```python
from build123d import *

# Parameters (mm, degrees)
ESTRUSIONE_ESTRUSIONE9_DEPTH = 50
SMUSSO1_SIZE                 = 0.75


with BuildPart() as part:
    # Schizzo16 → Estrusione-Estrusione9 (new body)
    with BuildSketch(Plane(origin=(0, 0, 0), x_dir=(0, 0, -1), z_dir=(1, 0, 0))):
        Polygon((0, 0), (5, 0), (5, 6), (43, 6), (43, 0), (48, 0), (48, 9), (0, 9), align=None)
    extrude(amount=ESTRUSIONE_ESTRUSIONE9_DEPTH)

    # Smusso1
    smusso1_edges = [part.edges().sort_by_distance(p)[0] for p in [
        (0, 4.5, 0),
        (50, 4.5, -48),
        (50, 4.5, 0),
        (0, 4.5, -48),
    ]]
    chamfer(smusso1_edges, length=SMUSSO1_SIZE)


solid = part.part
```
The listing builds one solid part. Answer for the finished solid, in the listing's coordinates (mm). A direction names the side the tool comes from. Coordinates: 2 decimals unless noted, no trailing zeros. Loops run counter-clockwise (first coordinate to the right, second up) from the corner with the lowest first, then second, coordinate; pieces in that order, holes last. Notation, with made-up numbers: (42, -16) - (78, -16) arc R18 ccw to (78, 11) - close; hole circle Ø5 at (76.5, 46.25). An arc over 180 degrees is marked (long way). Use a Markdown table: item, result. Add a question column.
1) The part is cut by section A-A, the plane y = 3. Give the vertices of the cut face in (x, z).
2) The part is cut by section C-C, the plane z = -19. Give the vertices of the cut face in (x, y), and give its area (3 significant figures).
3) Given pin 1 (5 mm diameter, centred on y = 5, z = -29, fed in from -X); pin 2 (3 mm diameter, centred on y = 3, z = -8, fed in from -X); pin 3 (11.5 mm diameter, centred on x = 20.5, z = -20, fed in from -Y), each flat-ended and moving along its own axis, determine where each tip first touches the part or whether it passes through.
4) The part is cut by section B-B, the plane x = 40. Give the vertices of the cut face in (y, z).
5) For faces 5 (the flat face through (25, 3, -43)), 6 (the flat face through (25, 4, -48)), determine the directions among +Z, -Z, +X, -X, +Y, -Y from which every point of the face is accessible in a straight line to the end or side of a thin tool.
6) The mould has two halves that part along Z. Classify faces 1 (the flat face through (25, 6, -24)), 2 (the flat face through (25, 5, 0)), 3 (the flat face through (25, 0, -2)), 4 (the flat face through (25, 3, -5)): released by +Z, released by -Z, zero draft, split by the parting line, or undercut.
7) Find the intervals of material crossed by line 1 (Z direction, x = 36, y = 1); line 2 (Y direction, x = 12, z = -30.5), in increasing order.
Here are the results:
| question | item | result |
|---|---|---|
| 1 | outline | (0, -47.25) - (0.75, -48) - (49.25, -48) - (50, -47.25) - (50, -43) - (0, -43) - close; (0, -5) - (50, -5) - (50, -0.75) - (49.25, 0) - (0.75, 0) - (0, -0.75) - close |
| 2 | outline | (0, 6) - (50, 6) - (50, 9) - (0, 9) - close |
| 2 | area | 150 mm^2 |
| 3 | pin 1 | stops at x = 0 |
| 3 | pin 2 | passes through |
| 3 | pin 3 | stops at y = 6 |
| 4 | outline | (0, -48) - (9, -48) - (9, 0) - (0, 0) - (0, -5) - (6, -5) - (6, -43) - (0, -43) - close |
| 5 | face 5 | +X, -X, -Y |
| 5 | face 6 | -Z, +X, -X, +Y, -Y |
| 6 | face 1 | undercut |
| 6 | face 2 | released by +Z |
| 6 | face 3 | zero draft |
| 6 | face 4 | undercut |
| 7 | line 1 | z = -48 to -43, -5 to 0 |
| 7 | line 2 | y = 6 to 9 |
